Verification items for this drawing (mm, ordinates from the low corner). Round coordinates to 2 decimals unless told otherwise and drop trailing zeros. Order: outer loops, then holes, each group sorted by start corner. A loop starts at its lowest first (then second) coordinate and runs counter-clockwise, first axis right, second up. Notation, with made-up numbers: (53, -29) - (96, -29) arc R14 cw to (96, -2) - close; hole circle Ø11 at (59, -38.75). An arc over 180 degrees is marked (long way). Return JSON: item names as keys, results as strings. Group by question number.
Q1. Gauge pin test, flat ends, axial feed: pin 1 Ø1 at (y, z) = (1, 40) entering from +X (1 decimal); pin 2 Ø5.5 at (x, z) = (90.17, 49.81) entering from -Y; pin 3 Ø2 at (y, z) = (3.5, 39) entering from +X; pin 4 Ø11.5 at (x, z) = (11.43, 51.79) entering from -Y. Record the tip position at first contact, or that the pin passes through.
Q2. Material ranges on line 1 along Z through (x, y) = (50.8, 3.75); line 2 along Z through (x, y) = (44, 5) (1 decimal); line 3 along X through (y, z) = (3.75, 41.5), recorded low to high.
Q3. Sectioned sample at A-A, the plane y = 2.5. Record the cut outline in (x, z).
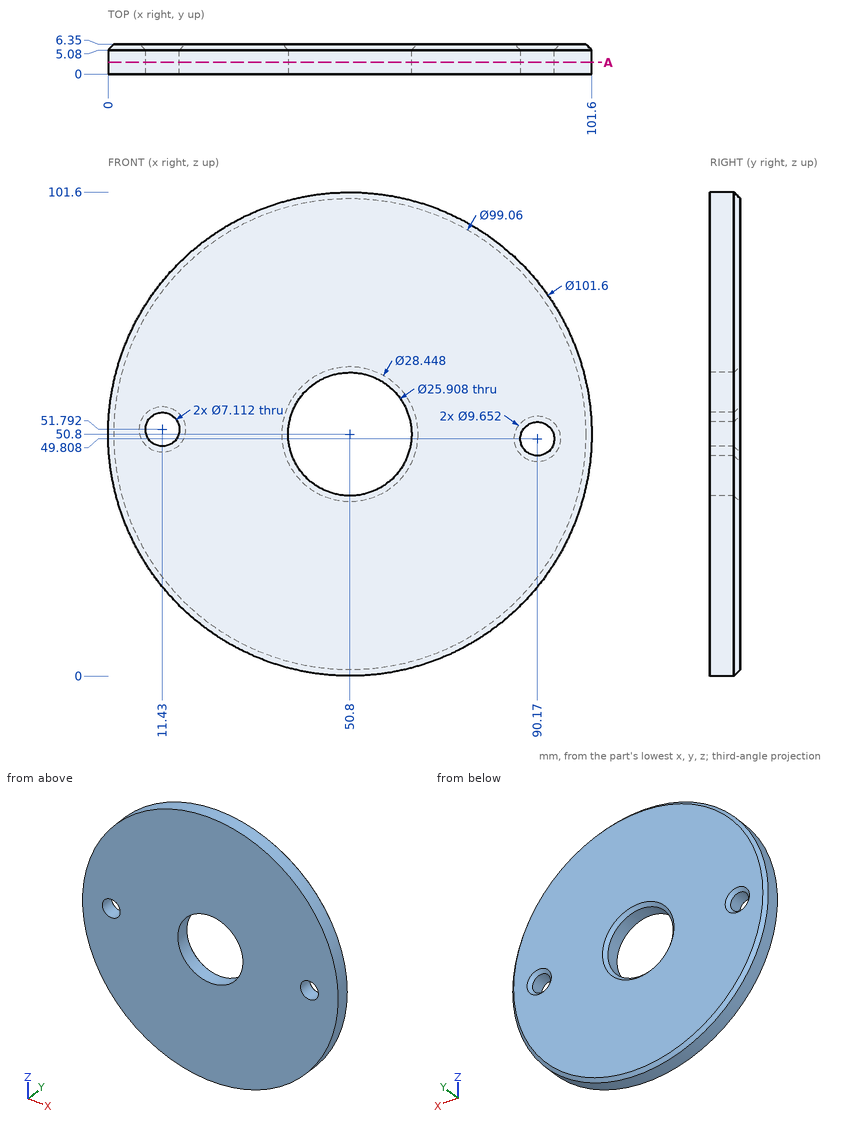
Reply:
{
 "1": {"pin 1": "x = 100.5", "pin 2": "through", "pin 3": "x = 100.44", "pin 4": "y = 0"},
 "2": {"line 1": "0 to 37.85, 63.75 to 101.6", "line 2": "0.5 to 39.8, 61.8 to 101.1", "line 3": "0.86 to 41.78, 59.82 to 100.74"},
 "3": {"outline": "circle Ø101.6 at (50.8, 50.8); hole circle Ø7.11 at (11.43, 51.79); hole circle Ø25.91 at (50.8, 50.8); hole circle Ø7.11 at (90.17, 49.81)"}
}
